Geometry check sheet. Reference: the model listing, model coordinates, mm. Coordinates: 2 decimals unless noted, no trailing zeros. Write each loop counter-clockwise with the first axis right and the second up, starting at its lowest first coordinate (ties: lowest second). Pieces come first, ordered by that corner, then holes. Notation, with made-up numbers: (2, 38) -> (55, 38) arc R16 cw to (55, 47) -> close; hole circle Ø8 at (22.25, 77). An arc over 180 degrees is marked (long way). Answer in a Markdown table with one row per item. Add a question column.
Q1. Section check A-A, the plane x = 0. Record the boundary of the cut face in (y, z) (3 decimals), and give its area (3 significant figures).
Q2. Section check C-C, the plane x = 32.5. Record the boundary of the cut face in (y, z).
Q3. Section check D-D, the plane z = -32.5. Record the boundary of the cut face in (x, y), and give its area (3 significant figures).
Q4. Section check B-B, the plane y = -3.75. Record the boundary of the cut face in (x, z) (3 decimals).
Q5. Thickness scan on line 1 (Z direction, x = 0, y = -5.25) (3 decimals); line 2 (Z direction, x = 1.5, y = -9.75); line 3 (X direction, y = -11, z = -58.5). Record the ranges inside material, lowest first.
Q6. Gauge pin test, flat ends, axial feed: P1, Ø1, axis at y = -9.5, z = 64, coming from the -X side; P2, Ø5, axis at x = -59.5, y = -11.5, coming from the +Z side; P3, Ø12, axis at x = -1, y = -15.5, coming from the -Z side. Record the tip position at first contact, or that the pin passes through.
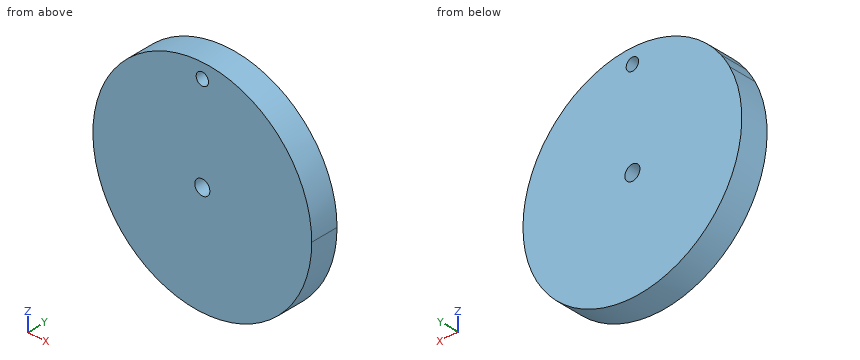
```python
from build123d import *

# Parameters (mm, degrees)
F0_R     = 101.6
F1_DEPTH = 25.4
F2_R     = 6.985
F3_DEPTH = 25.4
F5_DEPTH = 25.4
F6_R     = 5.7500810909
F7_DEPTH = 25.4


with BuildPart() as f1:
    # F0 (on Front) → F1 (new body)
    with BuildSketch(Plane.XZ):
        Circle(F0_R)
    extrude(amount=F1_DEPTH)

    # F2 (on face) → F3 (cut)
    with BuildSketch(Plane.XZ.offset(25.4)):
        Circle(F2_R)
    extrude(amount=-F3_DEPTH, mode=Mode.SUBTRACT)

    # F4 (on face) → F5 (cut)
    with BuildSketch(Plane.XZ.offset(25.4)):
        with BuildLine():
            ThreePointArc((-90.4125676958, 46.3478974998), (-86.5556978754, 53.2040521511), (-82.1799387694, 59.7412559615))
            Line((-82.1799387694, 59.7412559615), (-107.8644320369, 59.7412559615))
            Line((-107.8644320369, 59.7412559615), (-107.8644320369, 46.3478974998))
            Line((-107.8644320369, 46.3478974998), (-90.4125676958, 46.3478974998))
        make_face()
    extrude(amount=-F5_DEPTH, mode=Mode.SUBTRACT)

    # F6 (on face) → F7 (cut)
    with BuildSketch(Plane.XZ.offset(25.4)):
        with Locations((0, 87.9493951797)):
            Circle(F6_R)
    extrude(amount=-F7_DEPTH, mode=Mode.SUBTRACT)


solid = f1.part
```
Calculated:
| question | item | result |
|---|---|---|
| 1 | outline | (-25.4, -101.6) -> (0, -101.6) -> (0, -6.985) -> (-25.4, -6.985) -> close; (-25.4, 6.985) -> (0, 6.985) -> (0, 82.199) -> (-25.4, 82.199) -> close; (-25.4, 93.699) -> (0, 93.699) -> (0, 101.6) -> (-25.4, 101.6) -> close |
| 1 | area | 4,510 mm² |
| 2 | outline | (-25.4, -96.26) -> (0, -96.26) -> (0, 96.26) -> (-25.4, 96.26) -> close |
| 3 | outline | (-96.26, -25.4) -> (96.26, -25.4) -> (96.26, 0) -> (-96.26, 0) -> close |
| 3 | area | 4,890 mm² |
| 4 | outline | circle Ø203.2 at (0, 0); hole circle Ø13.97 at (0, 0); hole circle Ø11.5 at (0, 87.949) |
| 5 | line 1 | z = -101.6 to -6.985, 6.985 to 82.199, 93.699 to 101.6 |
| 5 | line 2 | z = -101.59 to -6.82, 6.82 to 82.4, 93.5 to 101.59 |
| 5 | line 3 | x = -83.07 to 83.07 |
| 6 | P1 | stops at x = -79.31 |
| 6 | P2 | stops at z = 84.1 |
| 6 | P3 | stops at z = -101.6 |
